Could you check a few things on this drawing? It's one solid part, dimensions in mm from its lowest x, y, z. Give positions to 0.01 mm unless a question says otherwise; leave off trailing zeros. Loops run counter-clockwise (first coordinate to the right, second up) from the corner with the lowest first, then second, coordinate; pieces in that order, holes last. Notation, with made-up numbers: M -32.75,-21.75 L -7.75,-21.75 A28 cw -7.75,8.25 Z; hole C 19.5,-36.5 d5. An arc over 180 degrees is marked long. Answer in a Markdown table with one row per item. Add a question column.
1. Thinking about a two-plate mould opening in X: for the marked faces 1, 2 and 3, which applies, released by +X, released by -X, zero draft, split by the parting line, or undercut?
2. I'm going to push flat-ended pins straight in: pin 1 Ø5 at (x, z) = (69.5, 6.5) entering from -Y; pin 2 Ø10 at (x, z) = (28, 24) entering from +Y; pin 3 Ø1 at (x, z) = (58.5, 7.5) entering from -Y. Where does each tip first touch, or does it pass through?
3. If we section it at B-B on z = 21: List the corners of the cut face in (x, y) for me.
4. If we section it at C-C on z = 26.25: List the corners of the cut face in (x, y) for me, then the cut area to 3 significant figures.
5. If we section it at A-A on y = 50: List the corners of the cut face in (x, z) for me, then the cut area to 3 significant figures.
6. I need wall thicknesses on line 1 along Y through (x, z) = (50, 22.25); line 2 along Z through (x, y) = (22.5, 14); line 3 along Y through (x, z) = (25.5, 27). Which ranges of each line are inside material? Lowest first, please. Write a range as from..to.
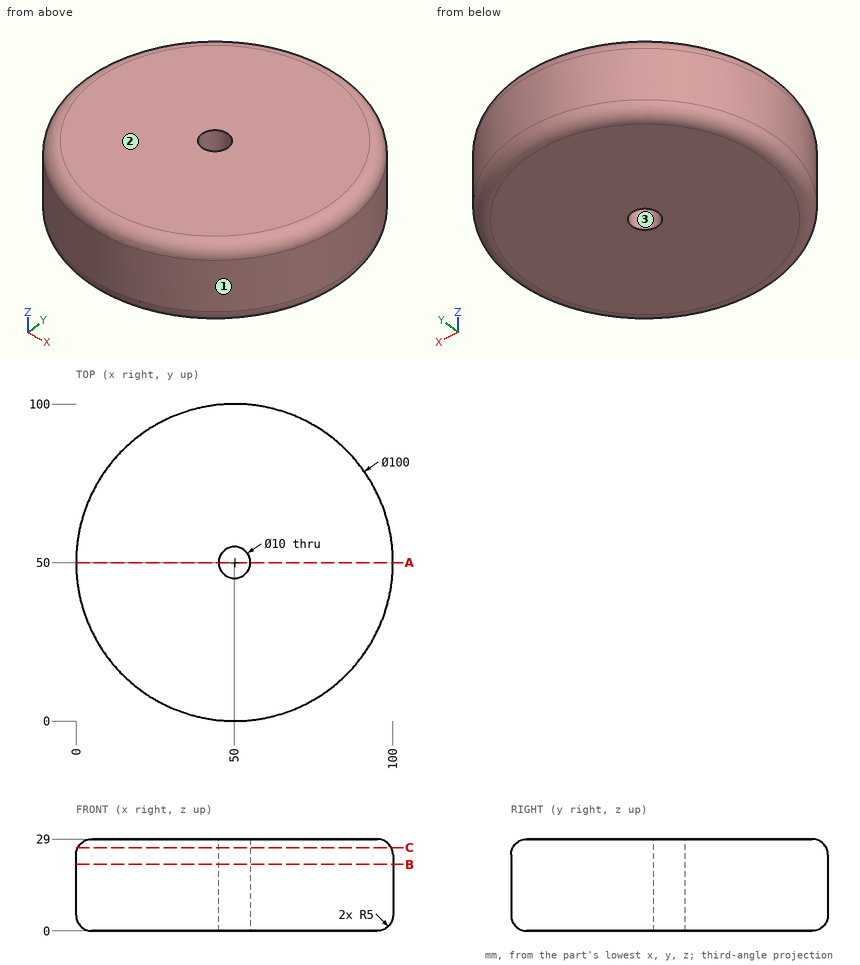
Results:
| question | item | result |
|---|---|---|
| 1 | face 1 | split by the parting line |
| 1 | face 2 | zero draft |
| 1 | face 3 | undercut |
| 2 | pin 1 | y = 2.98 |
| 2 | pin 2 | y = 97.02 |
| 2 | pin 3 | y = 0.64 |
| 3 | outline | C 50,50 d100; hole C 50,50 d10 |
| 4 | outline | C 50,50 d98.93; hole C 50,50 d10 |
| 4 | area | 7,610 mm2 |
| 5 | outline | M 0,5 A5 ccw 5,0 L 45,0 L 45,29 L 5,29 A5 ccw 0,24 Z; M 55,0 L 95,0 A5 ccw 100,5 L 100,24 A5 ccw 95,29 L 55,29 Z |
| 5 | area | 2,590 mm2 |
| 6 | line 1 | 0..45, 55..100 |
| 6 | line 2 | 0.01..28.99 |
| 6 | line 3 | 7.56..92.44 |
